Source: CAD feature listing. Evaluate the final solid. Frame: model axes, mm. Round coordinates to 2 decimals unless told otherwise and drop trailing zeros. Order: outer loops, then holes, each group sorted by start corner. A loop starts at its lowest first (then second) coordinate and runs counter-clockwise, first axis right, second up. Notation, with made-up numbers: (80, 30) -> (87, 30) arc R12 cw to (87, 38) -> close; hole circle Ø9 at (-22, -13). An arc over 180 degrees is marked (long way). Answer as CSV lines item,"result".
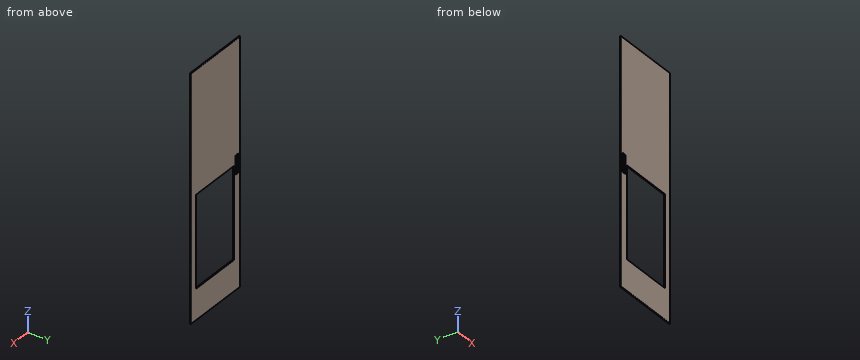
from build123d import *

# Parameters (mm, degrees)
F0_W     = 600
F0_H     = 2090
F0_W_2   = 463
F0_H_2   = 783
F0_W_3   = 35
F0_H_3   = 160
F1_DEPTH = 10
F2_R     = 4.99999


# Not quite as in the source:
# - a fillet or chamfer is up to 0.001 mm smaller than in the source, because OpenCascade refuses the exact size


with BuildPart() as f1:
    # F0 (on Front) → F1 (new body)
    with BuildSketch(Plane.XZ):
        Rectangle(F0_W, F0_H)
        with Locations((6.5, -388.5)):
            Rectangle(F0_W_2, F0_H_2, mode=Mode.SUBTRACT)
        with Locations((-262.5, 0)):
            Rectangle(F0_W_3, F0_H_3, mode=Mode.SUBTRACT)
    extrude(amount=F1_DEPTH)

    # F2 (radius 5 in the source; OpenCascade refuses exactly that, so slightly less here)
    f2_edges = [f1.edges().sort_by_distance(p)[0] for p in [
        (300, -5, 1045),
        (-300, -5, 1045),
        (-300, -5, -1045),
        (300, -5, -1045),
        (0, -10, -1045),
        (-300, -10, 0),
        (-300, 0, 0),
        (0, 0, -1045),
        (300, 0, 0),
        (300, -10, 0),
        (0, -10, 1045),
        (0, 0, 1045),
    ]]
    fillet(f2_edges, radius=F2_R)


solid = f1.part
1. Pin query (flat end, axial travel): pin 1 (6 mm diameter, centred on x = -103, y = -8.5, fed in from -Z); pin 2 (3 mm diameter, centred on y = -7, z = -319.5, fed in from -X); pin 3 (3 mm diameter, centred on y = -3, z = -13, fed in from +X). Return the tip coordinate at first contact, or that it passes through.
Results below:
pin 1,"z = -1044.97"
pin 2,"x = -299.97"
pin 3,"x = 299.97"
2. Line query: L1, parallel to Z at x = -16, y = -6.5; L2, parallel to Z at x = -99.5, y = -5.5; L3, parallel to X at y = -5.5, z = -343. Output: solid intervals per line, ascending. Write a range as [from, to].
Results below:
L1,"[-1044.77, -780], [3, 1044.77]"
L2,"[-1044.97, -780], [3, 1044.97]"
L3,"[-299.97, -225], [238, 299.97]"
3. Section query B-B on y = -8. Return loops of the section in (x, z), and give its area (3 significant figures).
Results below:
outline,"(-299, -1040) arc R4 ccw to (-295, -1044) -> (295, -1044) arc R4 ccw to (299, -1040) -> (299, 1040) arc R4 ccw to (295, 1044) -> (-295, 1044) arc R4 ccw to (-299, 1040) -> close; hole (-280, -80) -> (-245, -80) -> (-245, 80) -> (-280, 80) -> close; hole (-225, -780) -> (238, -780) -> (238, 3) -> (-225, 3) -> close"
area,"880,000 mm2"
